For this review, take the finished solid that the model builds, in its own axes (mm). Face numbers are marked on the shaded views. A direction names the side the tool comes from. Round coordinates to 2 decimals unless told otherwise and drop trailing zeros. Write each loop counter-clockwise with the first axis right and the second up, starting at its lowest first coordinate (ties: lowest second). Pieces come first, ordered by that corner, then holes. Notation, with made-up numbers: (32.25, 64) - (87.25, 64) arc R19 ccw to (87.25, 74) - close; hole circle Ø4 at (30.25, 4.5). An arc over 180 degrees is marked (long way). One line per item, written item: value. Start each with the question number.
Q1. Add section B-B on y = -3.5. Write out the cut boundary in (x, z), and give its area (3 significant figures).
Q2. Clearance check with flat-ended pins moving along their axes: pin 1 Ø2.5 at (x, z) = (25, -52) entering from +Y; pin 2 Ø6.5 at (x, z) = (25.5, -51) entering from -Y; pin 3 Ø4 at (x, y) = (22, -4) entering from -Z. State where each tip first meets the part, or that it passes through.
Q3. Add section A-A on x = -25.5. Write out the cut boundary in (y, z), and give its area (3 significant figures).
Q4. For probe 1 along X at (y, z) = (2.7, -51); probe 2 along X at (y, z) = (-2.6, -47); probe 3 along Y at (x, z) = (3.5, 8.5), list the stretches that pass through material, from the lowest coordinate up.
Q5. Add section C-C on z = -23. Write out the cut boundary in (x, y).
Q6. Add section D-D on z = -47. Write out the cut boundary in (x, y).
Q7. Tool access review of the marked faces 1 and 2: name each direction out of +Z, -Z, +X, -X, +Y, -Y from which nothing blocks a thin tool from reaching the whole face with its end or side.
```python
from build123d import *

# Parameters (mm, degrees)
CROQUIS1_W              = 57
CROQUIS1_H              = 108
SALIENTE_EXTRUIR1_DEPTH = 3
CROQUIS2_R              = 1.5
CORTAR_EXTRUIR1_DEPTH   = 3
CROQUIS3_R              = 2.5
CORTAR_EXTRUIR2_DEPTH   = 1
CROQUIS7_R              = 3.5
CROQUIS7_R_2            = 1.5
SALIENTE_EXTRUIR2_DEPTH = 5
CORTAR_EXTRUIR3_DEPTH   = 4


with BuildPart() as part:
    # Croquis1 → Saliente-Extruir1 (new body)
    with BuildSketch(Plane(origin=(0, 0, 0), x_dir=(1, 0, 0), z_dir=(0, 1, 0))):
        Rectangle(CROQUIS1_W, CROQUIS1_H)
    extrude(amount=SALIENTE_EXTRUIR1_DEPTH)

    # Croquis2 → Cortar-Extruir1 (cut)
    with BuildSketch(Plane(origin=(0, 3, 0), x_dir=(1, 0, 0), z_dir=(0, 1, 0))):
        with Locations(Location((-25.5, 51, 0), (0, 0, 270))):
            Circle(CROQUIS2_R)
        with Locations(Location((25.5, 51, 0), (0, 0, 270))):
            Circle(CROQUIS2_R)
        with Locations(Location((25.5, -51, 0), (0, 0, 270))):
            Circle(CROQUIS2_R)
        with Locations(Location((-25.5, -51, 0), (0, 0, 270))):
            Circle(CROQUIS2_R)
    extrude(amount=-CORTAR_EXTRUIR1_DEPTH, mode=Mode.SUBTRACT)

    # Croquis3 → Cortar-Extruir2 (cut)
    with BuildSketch(Plane(origin=(0, 3, 0), x_dir=(1, 0, 0), z_dir=(0, 1, 0))):
        with Locations(Location((-25.5, 51, 0), (0, 0, 270))):
            Circle(CROQUIS3_R)
        with Locations(Location((25.5, 51, 0), (0, 0, 270))):
            Circle(CROQUIS3_R)
        with Locations(Location((25.5, -51, 0), (0, 0, 270))):
            Circle(CROQUIS3_R)
        with Locations(Location((-25.5, -51, 0), (0, 0, 270))):
            Circle(CROQUIS3_R)
    extrude(amount=-CORTAR_EXTRUIR2_DEPTH, mode=Mode.SUBTRACT)

    # Croquis7 → Saliente-Extruir2 (add)
    # profile 1 of 4: a face of its own
    with BuildSketch(Plane.XZ):
        with Locations(Location((-17, 47, 0), (0, 0, 90))):
            Circle(CROQUIS7_R)
        with Locations(Location((-17, 47, 0), (0, 0, 270))):
            Circle(CROQUIS7_R_2, mode=Mode.SUBTRACT)
    # profile 2 of 4: a face of its own
    with BuildSketch(Plane.XZ):
        with Locations(Location((17, 47, 0), (0, 0, 90))):
            Circle(CROQUIS7_R)
        with Locations(Location((17, 47, 0), (0, 0, 270))):
            Circle(CROQUIS7_R_2, mode=Mode.SUBTRACT)
    # profile 3 of 4: a face of its own
    with BuildSketch(Plane.XZ):
        with Locations(Location((17, -47, 0), (0, 0, 90))):
            Circle(CROQUIS7_R)
        with Locations(Location((17, -47, 0), (0, 0, 270))):
            Circle(CROQUIS7_R_2, mode=Mode.SUBTRACT)
    # profile 4 of 4: a face of its own
    with BuildSketch(Plane.XZ):
        with Locations(Location((-17, -47, 0), (0, 0, 90))):
            Circle(CROQUIS7_R)
        with Locations(Location((-17, -47, 0), (0, 0, 270))):
            Circle(CROQUIS7_R_2, mode=Mode.SUBTRACT)
    extrude(amount=SALIENTE_EXTRUIR2_DEPTH)

    # Croquis9 → Cortar-Extruir3 (cut)
    with BuildSketch(Plane(origin=(0, 3, 0), x_dir=(1, 0, 0), z_dir=(0, 1, 0))):
        with BuildLine():
            Line((14.5, 33), (14.5, 19))
            ThreePointArc((14.5, 19), (18.5, 15), (22.5, 19))
            Line((22.5, 19), (22.5, 33))
            ThreePointArc((22.5, 33), (18.5, 37), (14.5, 33))
        make_face()
    extrude(amount=-CORTAR_EXTRUIR3_DEPTH, mode=Mode.SUBTRACT)


solid = part.part
```
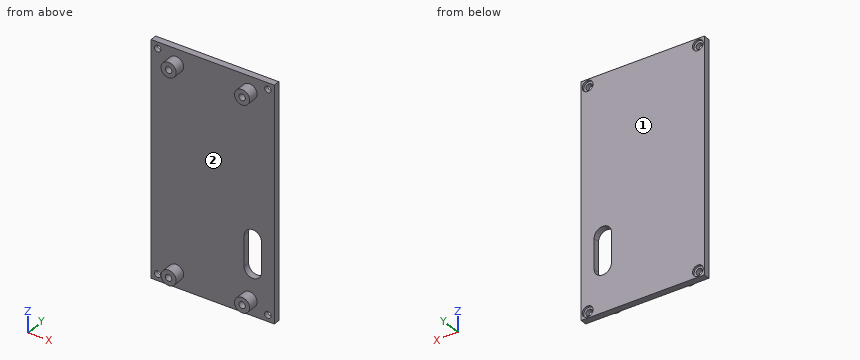
Result set:
1. outline: circle Ø7 at (-17, -47); circle Ø7 at (-17, 47); circle Ø7 at (17, -47); circle Ø7 at (17, 47); hole circle Ø3 at (-17, -47); hole circle Ø3 at (-17, 47); hole circle Ø3 at (17, -47); hole circle Ø3 at (17, 47)
1. area: 126 mm^2
2. pin 1: stops at y = 2
2. pin 2: stops at y = 0
2. pin 3: stops at z = -48.8
3. outline: (0, -54) - (3, -54) - (3, -53.5) - (2, -53.5) - (2, -52.5) - (0, -52.5) - close; (0, -49.5) - (2, -49.5) - (2, -48.5) - (3, -48.5) - (3, 48.5) - (2, 48.5) - (2, 49.5) - (0, 49.5) - close; (0, 52.5) - (2, 52.5) - (2, 53.5) - (3, 53.5) - (3, 54) - (0, 54) - close
3. area: 302 mm^2
4. probe 1: x = -28.5 to -28, -23 to 23, 28 to 28.5
4. probe 2: x = -20.5 to -18.5, -15.5 to -13.5, 13.5 to 15.5, 18.5 to 20.5
4. probe 3: y = 0 to 3
5. outline: (-28.5, 0) - (14.5, 0) - (14.5, 3) - (-28.5, 3) - close; (22.5, 0) - (28.5, 0) - (28.5, 3) - (22.5, 3) - close
6. outline: (-28.5, 0) - (-20.5, 0) - (-20.5, -5) - (-18.5, -5) - (-18.5, 0) - (-15.5, 0) - (-15.5, -5) - (-13.5, -5) - (-13.5, 0) - (13.5, 0) - (13.5, -5) - (15.5, -5) - (15.5, 0) - (18.5, 0) - (18.5, -5) - (20.5, -5) - (20.5, 0) - (28.5, 0) - (28.5, 3) - (-28.5, 3) - close
7. face 1: +Z, -Z, +X, -X, +Y
7. face 2: -Y
